Geometry: final body of the model. Coordinates: model frame, mm. A direction names the side the tool comes from. Coordinates: 2 decimals unless noted, no trailing zeros. Write each loop counter-clockwise with the first axis right and the second up, starting at its lowest first coordinate (ties: lowest second). Pieces come first, ordered by that corner, then holes.
from build123d import *

# Parameters (mm, degrees)
F1_DEPTH    = 250
F2_W        = 38
F2_H        = 13.3740238536
F3_DEPTH    = 1200
F4_T1_DEPTH = 509.3674969976
F5_R        = 9
F6_R        = 1
F8_DEPTH    = 500.001


# Not quite as in the source:
# - a fillet or chamfer that OpenCascade refuses, or shapes differently, is made with other operations: its cross-section is extruded or revolved along the edge and cut away or added


with BuildPart() as f1:
    # F0 (on Front) → F1 (new body, symmetric)
    with BuildSketch(Plane.XZ):
        with BuildLine():
            Line((-57.5, 2.6740238536), (-40.1794919243, -7.3259761464))
            ThreePointArc((-40.1794919243, -7.3259761464), (0, -3.248431288), (40.1794919243, -7.3259761464))
            Line((40.1794919243, -7.3259761464), (57.5, 2.6740238536))
            Line((57.5, 2.6740238536), (57.5, 6.6740238536))
            Line((57.5, 6.6740238536), (45.5824640741, 16.6740238536))
            Line((45.5824640741, 16.6740238536), (22.5, 16.6740238536))
            Line((22.5, 16.6740238536), (22.5, 15.3740238536))
            Line((22.5, 15.3740238536), (0, 15.3740238536))
            Line((0, 15.3740238536), (-22.5, 15.3740238536))
            Line((-22.5, 15.3740238536), (-22.5, 16.6740238536))
            Line((-22.5, 16.6740238536), (-45.5824640741, 16.6740238536))
            Line((-45.5824640741, 16.6740238536), (-57.5, 6.6740238536))
            Line((-57.5, 6.6740238536), (-57.5, 2.6740238536))
        make_face()
    extrude(amount=F1_DEPTH, both=True)

    # F2 (on face) → F3 (cut)
    with BuildSketch(Plane.XZ.offset(250)):
        with Locations((0, 6.6870119268)):
            Rectangle(F2_W, F2_H)
    extrude(amount=-F3_DEPTH, mode=Mode.SUBTRACT)

    # F4: fillet of radius 2 on 2 edges, made by hand

    # F4_s2 → F4_t1 (cut)
    with BuildSketch(Plane.XZ.offset(-254.6837484988)):
        with BuildLine():
            ThreePointArc((-24.3734993995, 16.6740238536), (-23.2333239744, 16.3171915261), (-22.5, 15.3740238536))
            Line((-22.5, 15.3740238536), (-22.5, 16.6740238536))
            Line((-22.5, 16.6740238536), (-24.3734993995, 16.6740238536))
        make_face()
        with BuildLine():
            ThreePointArc((24.3734993995, 16.6740238536), (23.2333239744, 16.3171915261), (22.5, 15.3740238536))
            Line((22.5, 15.3740238536), (22.5, 16.6740238536))
            Line((22.5, 16.6740238536), (24.3734993995, 16.6740238536))
        make_face()
    extrude(amount=F4_T1_DEPTH, mode=Mode.SUBTRACT)

    # F5
    f5_edges = [f1.edges().sort_by_distance(p)[0] for p in [
        (45.582464, 0, 16.674024),
        (40.179492, 0, -7.325976),
        (-45.582464, 0, 16.674024),
        (-40.179492, 0, -7.325976),
    ]]
    fillet(f5_edges, radius=F5_R)

    # F6
    f6_edges = [f1.edges().sort_by_distance(p)[0] for p in [
        (-57.5, 0, 6.674024),
        (-57.5, 0, 2.674024),
        (57.5, 0, 6.674024),
        (57.5, 0, 2.674024),
    ]]
    fillet(f6_edges, radius=F6_R)

    # F7 (on face) → F8 (cut, through all)
    with BuildSketch(Plane.XZ.offset(250)):
        with BuildLine():
            ThreePointArc((-42.102269028, -3.9064590428), (-39.7790673217, -4.7446540804), (-37.3093701512, -4.7238460325))
            ThreePointArc((-37.3093701512, -4.7238460325), (-29.178978452, -3.3669982622), (-20.9999997169, -2.3429807302))
            Line((-20.9999997169, -2.3429807302), (-20.9999997169, 13.3740240708))
            Line((-20.9999997169, 13.3740240708), (-22.500000096, 13.3740240708))
            ThreePointArc((-22.500000096, 13.3740240708), (-23.2333241124, 14.3171915037), (-24.3734993995, 14.6740237251))
            Line((-24.3734993995, 14.6740237251), (-42.3067319657, 14.6740237251))
            ThreePointArc((-42.3067319657, 14.6740237251), (-44.700872925, 14.2518720783), (-46.8062451509, 13.036334857))
            Line((-46.8062451509, 13.036334857), (-55.4999998715, 5.7414084774))
            Line((-55.4999998715, 5.7414084774), (-55.4999998715, 3.8287244662))
            Line((-55.4999998715, 3.8287244662), (-42.102269028, -3.9064590428))
        make_face()
        with BuildLine():
            ThreePointArc((24.3734993995, 14.6740237251), (23.2333241124, 14.3171915037), (22.500000096, 13.3740240708))
            Line((22.500000096, 13.3740240708), (20.9999997169, 13.3740240708))
            Line((20.9999997169, 13.3740240708), (20.9999997169, -2.3429807302))
            ThreePointArc((20.9999997169, -2.3429807302), (29.178978452, -3.3669982622), (37.3093701512, -4.7238460325))
            ThreePointArc((37.3093701512, -4.7238460325), (39.7790673217, -4.7446540804), (42.102269028, -3.9064590428))
            Line((42.102269028, -3.9064590428), (55.4999998715, 3.8287244662))
            Line((55.4999998715, 3.8287244662), (55.4999998715, 5.7414084774))
            Line((55.4999998715, 5.7414084774), (46.8062451509, 13.036334857))
            ThreePointArc((46.8062451509, 13.036334857), (44.700872925, 14.2518720783), (42.3067319657, 14.6740237251))
            Line((42.3067319657, 14.6740237251), (24.3734993995, 14.6740237251))
        make_face()
    extrude(amount=-F8_DEPTH, mode=Mode.SUBTRACT)


solid = f1.part
Item 1: Pin query (flat end, axial travel): pin 1 (6 mm diameter, centred on x = -20, y = -173, fed in from -Z); pin 2 (5.5 mm diameter, centred on x = -31, y = -60.5, fed in from -Z); pin 3 (19 mm diameter, centred on x = -6.5, y = -65, fed in from +Z). Return the tip coordinate at first contact, or that it passes through.
Derived:
pin 1: stops at z = -4.58
pin 2: stops at z = -6.12
pin 3: stops at z = 15.37
Item 2: Section A-A, the plane x = 30. Output: boundary loops of the cut face in (y, z), plus the area to 3 significant figures.
Derived:
outline: (-250, -5.51) - (250, -5.51) - (250, -3.49) - (-250, -3.49) - close; (-250, 14.67) - (250, 14.67) - (250, 16.67) - (-250, 16.67) - close
area: 2,010 mm2
Item 3: Pull-direction query (X, two-part tool) for faces 4 (the flat face through (-33, -4, 14.674)), 5 (the flat face through (-51.09, -3.5, 9.44)), 6 (the flat face through (-33, -4, 16.674)), 7 (the flat face through (52.7, -3.5, 10.7)); classes: released by +X, released by -X, zero draft, split by the parting line, or undercut.
Derived:
face 4: undercut
face 5: undercut
face 6: zero draft
face 7: released by +X
Item 4: Set-up query: faces 1 (the flat face through (-21, -4, 5)), 2 (the flat face through (-0.3, 250, -0.3)), 3 (the flat face through (0, -4, 15.374)). Return all of +Z, -Z, +X, -X, +Y, -Y with unobstructed straight access to the full face (end or side cutting, diameter ignored); none if empty.
Derived:
face 1: +Y, -Y
face 2: +Z, -Z, +X, -X, +Y
face 3: +Z, +Y, -Y
Item 5: Section B-B, the plane y = 212. State how many separate pieces and enclosed holes the cut face has, plus the area to 3 significant figures.
Derived:
separate pieces: 1
enclosed holes: 3
area: 608 mm2
Item 6: Material intervals for probe 1 along X at (y, z) = (-51.5, 5.5); probe 2 along Z at (x, y) = (-16, -190); probe 3 along X at (y, z) = (171, 1.25), sorted ascending.
Derived:
probe 1: x = -57.5 to -55.5, -21 to -19, 19 to 21, 55.5 to 57.5
probe 2: z = -3.89 to 0, 13.37 to 15.37
probe 3: x = -55.03 to -51.03, -21 to -19, 19 to 21, 51.03 to 55.03
